Build history of the part. All positions in model axes, mm. Face numbers are marked on the shaded views. Round coordinates to 2 decimals unless told otherwise and drop trailing zeros. Order: outer loops, then holes, each group sorted by start corner. A loop starts at its lowest first (then second) coordinate and runs counter-clockwise, first axis right, second up. Notation, with made-up numbers: M -32.75,-14.75 L -21.75,-14.75 A33 ccw -21.75,21.25 Z; hole C 16,-20.75 d9. An arc over 180 degrees is marked long. Use CSV: the item, a comma, the result in double quotes.
from build123d import *

# Parameters (mm, degrees)
SKETCH1_R           = 32.5
SKETCH1_R_2         = 17.5
SKETCH1_R_3         = 12.5
SKETCH1_R_4         = 8
BOSS_EXTRUDE1_DEPTH = 5
SKETCH2_R           = 1.5
CUT_EXTRUDE1_DEPTH  = 10
SKETCH3_R           = 8
SKETCH3_R_2         = 5.5
BOSS_EXTRUDE3_DEPTH = 30


with BuildPart() as part:
    # Sketch1 → Boss-Extrude1 (new body)
    with BuildSketch(Plane(origin=(0, 0, 0), x_dir=(1, 0, 0), z_dir=(0, 1, 0))):
        Circle(SKETCH1_R)
        Circle(SKETCH1_R_2, mode=Mode.SUBTRACT)
        Circle(SKETCH1_R_2)
        Circle(SKETCH1_R_3, mode=Mode.SUBTRACT)
        Circle(SKETCH1_R_3)
        Circle(SKETCH1_R_4, mode=Mode.SUBTRACT)
    extrude(amount=BOSS_EXTRUDE1_DEPTH)

    # Sketch2 → Cut-Extrude1 (cut)
    with BuildSketch(Plane(origin=(0, 0, 0), x_dir=(1, 0, 0), z_dir=(0, 1, 0))):
        with Locations((-7.247844507, 7.247844507)):
            Circle(SKETCH2_R)
        with Locations((7.247844507, 7.247844507)):
            Circle(SKETCH2_R)
        with Locations((7.247844507, -7.247844507)):
            Circle(SKETCH2_R)
        with Locations((-7.247844507, -7.247844507)):
            Circle(SKETCH2_R)
    extrude(amount=CUT_EXTRUDE1_DEPTH, mode=Mode.SUBTRACT)

    # Sketch3 → Boss-Extrude3 (add)
    with BuildSketch(Plane(origin=(0, 0, 0), x_dir=(1, 0, 0), z_dir=(0, 1, 0))):
        Circle(SKETCH3_R)
        Circle(SKETCH3_R_2, mode=Mode.SUBTRACT)
    extrude(amount=BOSS_EXTRUDE3_DEPTH)


solid = part.part
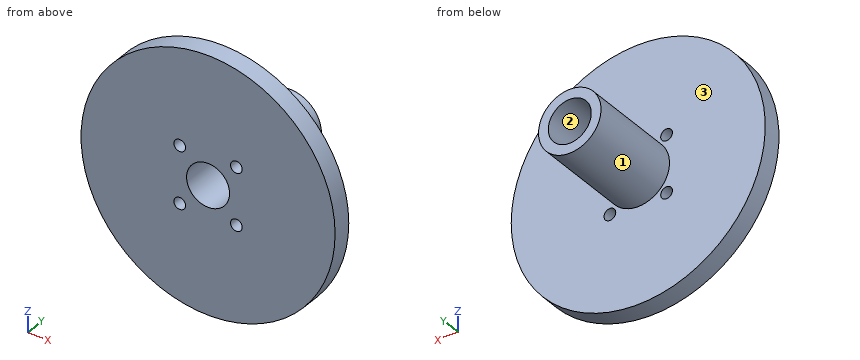
(1) Cut at A-A, the plane z = 0. Give the cut face in (x, y).
Answer block:
outline,"M -32.5,0 L -5.5,0 L -5.5,30 L -8,30 L -8,5 L -32.5,5 Z; M 5.5,0 L 32.5,0 L 32.5,5 L 8,5 L 8,30 L 5.5,30 Z"
(2) Cut at C-C, the plane y = 14.5. Give the cut face in (x, z).
Answer block:
outline,"C 0,0 d16; hole C 0,0 d11"
(3) Two-plate mould, pull along Z, no slides. Class the marked faces 1, 2 and 3: released by +Z, released by -Z, zero draft, split by the parting line, or undercut.
Answer block:
face 1,"split by the parting line"
face 2,"undercut"
face 3,"zero draft"
(4) Cut at B-B, the plane x = 1.5. Give the cut face in (y, z).
Answer block:
outline,"M 0,-32.47 L 5,-32.47 L 5,-7.86 L 30,-7.86 L 30,-5.29 L 0,-5.29 Z; M 0,5.29 L 30,5.29 L 30,7.86 L 5,7.86 L 5,32.47 L 0,32.47 Z"
(5) Drop flat-ended pins along their axis: pin 1 (2 mm diameter, centred on x = -0.5, z = -11, fed in from +Y); pin 2 (12 mm diameter, centred on y = 18.5, z = 6, fed in from +X); pin 3 (12 mm diameter, centred on x = -11, y = 16, fed in from +Z) (3 decimals). Give the stop position or say it passes through.
Answer block:
pin 1,"stops at y = 5"
pin 2,"stops at x = 8"
pin 3,"stops at z = 6.245"
(6) Wall check: line 1 (X direction, y = 19.75, z = 0); line 2 (Y direction, x = 8, z = -4). Give the ranges that are in metal, low to high. Write a range as from..to.
Answer block:
line 1,"x = -8..-5.5, 5.5..8"
line 2,"y = 0..5"
(7) Cut at D-D, the plane z = -19.5. Give the cut face in (x, y), and give its area (3 significant figures).
Answer block:
outline,"M -26,0 L 26,0 L 26,5 L -26,5 Z"
area,"260 mm²"
